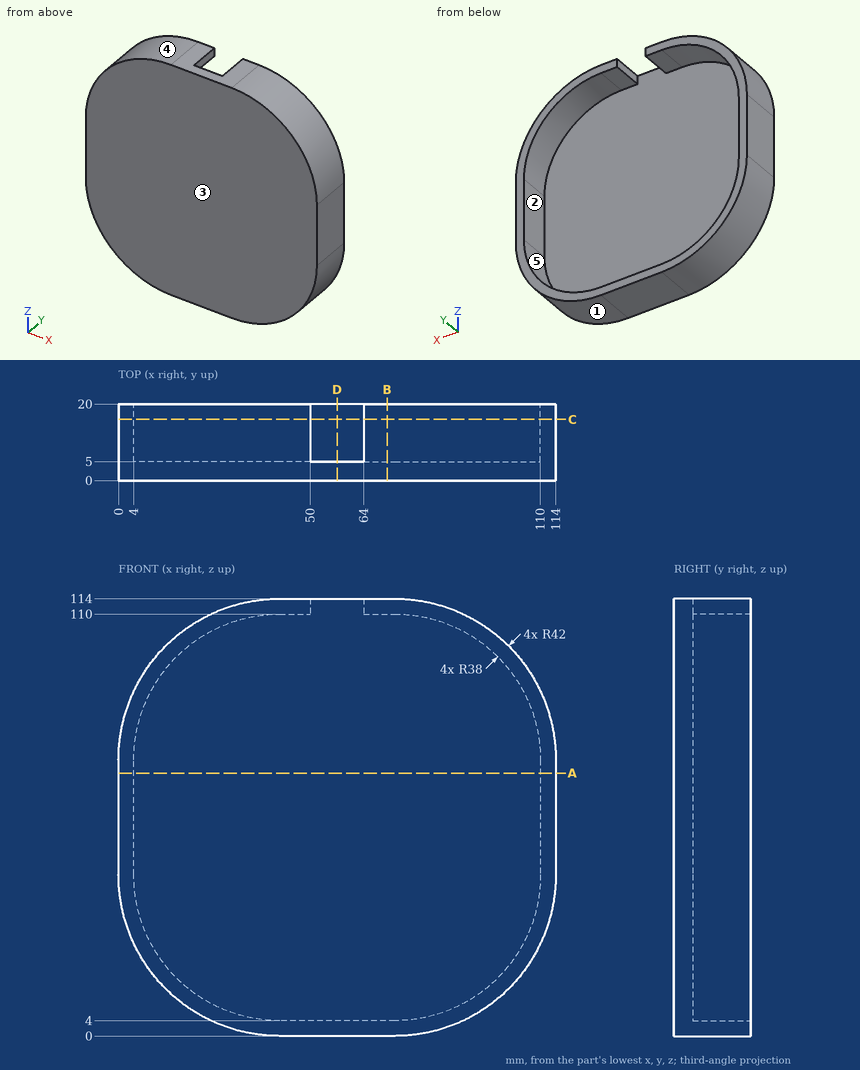
Design review of the part shown in the three views and the two pictorial views. Dimensions are in mm from the part's minimum x, y and z. A direction names the side the tool comes from. Round coordinates to 2 decimals unless told otherwise and drop trailing zeros. Write each loop counter-clockwise with the first axis right and the second up, starting at its lowest first coordinate (ties: lowest second). Pieces come first, ordered by that corner, then holes. Notation, with made-up numbers: (52, -8) - (102, -8) arc R6 cw to (102, 3) - close; hole circle Ø11 at (-16.75, -31.5). An arc over 180 degrees is marked (long way). Return JSON: item names as keys, results as strings. Group by question number.
Item 1: We need section C-C on y = 16. Write out the cut boundary in (x, z), and give its area (3 significant figures).
Item 2: We need section B-B on x = 70. Write out the cut boundary in (y, z), and give its area (3 significant figures).
Item 3: We need section A-A on z = 68.5. Write out the cut boundary in (x, y), and give its area (3 significant figures).
Item 4: Insertion check: P1, Ø5, axis at x = 87.5, y = 15, coming from the +Z side; P2, Ø3, axis at y = 13, z = 111, coming from the -X side; P3, Ø10, axis at x = 30.5, y = 13.5, coming from the +Z side; P4, Ø4, axis at x = 67.5, y = 12.5, coming from the -Z side. Each pin has a flat end and moves straight along its axis. Give the tip position at first contact, or say it passes through.
Item 5: We need section D-D on x = 57. Write out the cut boundary in (y, z), and give its area (3 significant figures).
Item 6: The part is to be moulded in two halves that separate along Z. For the marked faces 3, 4 and 5, say which applies: pulls with the +Z half, pulls with the -Z half, needs draft (parallel to the pull), parting line crosses it, or undercut.
Item 7: Machinability: for the marked faces 1 and 2, which of the approach directions +Z, -Z, +X, -X, +Y, -Y give a long, thin tool a straight path to every point of the face, cutting with its end or side? Answer none if there is none.
Item 8: For probe 1 along Z at (x, y) = (45.5, 16.5); probe 2 along Y at (x, z) = (94, 77), list the stretches that pass through material, from the lowest coordinate up. Write a range as [from, to].
Model answer:
{
 "1": {"outline": "(0, 42) arc R42 ccw to (42, 0) - (72, 0) arc R42 ccw to (114, 42) - (114, 72) arc R42 ccw to (72, 114) - (64, 114) - (64, 110) - (72, 110) arc R38 cw to (110, 72) - (110, 42) arc R38 cw to (72, 4) - (42, 4) arc R38 cw to (4, 42) - (4, 72) arc R38 cw to (42, 110) - (50, 110) - (50, 114) - (42, 114) arc R42 ccw to (0, 72) - close", "area": "1,430 mm²"},
 "2": {"outline": "(0, 0) - (20, 0) - (20, 4) - (5, 4) - (5, 110) - (20, 110) - (20, 114) - (0, 114) - close", "area": "690 mm²"},
 "3": {"outline": "(0, 0) - (114, 0) - (114, 20) - (110, 20) - (110, 5) - (4, 5) - (4, 20) - (0, 20) - close", "area": "690 mm²"},
 "4": {"P1": "stops at z = 111.94", "P2": "stops at x = 23.09", "P3": "stops at z = 113.49", "P4": "stops at z = 0"},
 "5": {"outline": "(0, 0) - (20, 0) - (20, 4) - (5, 4) - (5, 114) - (0, 114) - close", "area": "630 mm²"},
 "6": {"face 3": "needs draft", "face 4": "pulls with the +Z half", "face 5": "undercut"},
 "7": {"face 1": "-Z, +X, +Y, -Y", "face 2": "+Y"},
 "8": {"probe 1": "z = [0, 4], [110, 114]", "probe 2": "y = [0, 5]"}
}
